The model under review builds one solid part; all positions refer to its coordinate system, in mm. A direction names the side the tool comes from. Coordinates: 2 decimals unless noted, no trailing zeros. Write each loop counter-clockwise with the first axis right and the second up, starting at its lowest first coordinate (ties: lowest second). Pieces come first, ordered by that corner, then holes. Notation, with made-up numbers: M 33,75.5 L 56,75.5 A12 ccw 56,92.5 Z; hole C 29.25,33.5 d5. An arc over 180 degrees is marked long. Answer as a JSON object with one key per item and string values.
```python
from build123d import *

# Parameters (mm, degrees)
CHANFREIN1_SIZE              = 0.5
ENL_V_MAT_EXTRU_1_DEPTH      = 8.95
ENL_V_MAT_EXTRU_1_DEPTH_BACK = 8.95


with BuildPart() as part:
    # Esquisse1 → Base-Révolution (revolve)
    with BuildSketch(Plane.XY, mode=Mode.PRIVATE) as base_r_volution_sk:
        with BuildLine():
            Line((0, 65), (4, 65))
            Line((4, 65), (4, 49))
            Line((4, 49), (6, 49))
            Line((6, 49), (6, 27))
            Line((6, 27), (7.95, 27))
            Line((7.95, 27), (7.95, 7.95))
            ThreePointArc((7.95, 7.95), (5.62149891, 2.32850109), (0, 0))
            Line((0, 0), (0, 65))
        make_face()
    revolve(base_r_volution_sk.sketch.rotate(Axis((0, -9.281443849, 0), (0, 1, 0)), 90), axis=Axis((0, -9.281443849, 0), (0, 1, 0)))  # turned: the seam where the file's is

    # Chanfrein1
    chanfrein1_edges = [part.edges().sort_by_distance(p)[0] for p in [
        (0, 65, 4),
    ]]
    chamfer(chanfrein1_edges, length=CHANFREIN1_SIZE)

    # Esquisse2 → Enlèv. mat.-Extru.1 (cut, two sides)
    with BuildSketch(Plane.XY) as enl_v_mat_extru_1_sk:
        Polygon((14.617538198, 1), (14.617538198, 10), (3.65, 10), (7.95, 21.8), (23.946768439, 21.8), (23.946768439, -11.083879123), (-11.532407151, -11.083879123), (-11.532407151, 1), align=None)
    extrude(amount=ENL_V_MAT_EXTRU_1_DEPTH, mode=Mode.SUBTRACT)
    extrude(enl_v_mat_extru_1_sk.sketch, amount=-ENL_V_MAT_EXTRU_1_DEPTH_BACK, mode=Mode.SUBTRACT)


solid = part.part
```
(1) Add section A-A on x = 0. Give the boundary of the cut face in (y, z), and give its area (3 significant figures).
Results list:
{"outline": "M 1,-3.86 A7.95 ccw 7.95,-7.95 L 27,-7.95 L 27,-6 L 49,-6 L 49,-4 L 64.5,-4 L 65,-3.5 L 65,3.5 L 64.5,4 L 49,4 L 49,6 L 27,6 L 27,7.95 L 7.95,7.95 A7.95 ccw 1,3.86 Z", "area": "789 mm²"}
(2) Add section C-C on y = 51.5. Give the boundary of the cut face in (x, z), and give its area (3 significant figures).
Results list:
{"outline": "C 0,0 d8", "area": "50.3 mm²"}
(3) For faces 4 (the face through (0, 65, 0)), 5 (the face through (-1.802, 37.846, -5.723)), list the 3-axis set-ups (+Z, -Z, +X, -X, +Y, -Y) from which the entire face can be reached by the end or side of a thin tool; tool diameter is ignored.
Results list:
{"face 4": "+Z, -Z, +X, -X, +Y", "face 5": "+Y"}
(4) Add section B-B on z = 0. Give the boundary of the cut face in (x, y), and give its area (3 significant figures).
Results list:
{"outline": "M -7.95,7.95 A7.95 ccw -3.86,1 L 3.86,1 A7.95 ccw 7.95,7.95 L 7.95,10 L 3.65,10 L 7.95,21.8 L 7.95,27 L 6,27 L 6,49 L 4,49 L 4,64.5 L 3.5,65 L -3.5,65 L -4,64.5 L -4,49 L -6,49 L -6,27 L -7.95,27 Z", "area": "763 mm²"}
(5) Wall thickness on line 1 along Z through (x, y) = (-5.25, 31); line 2 along X through (y, z) = (57, 0.75); line 3 along X through (y, z) = (22, 0.25): over which ranges is each line inside the solid? List them lowest first. Write a range as from..to.
Results list:
{"line 1": "-2.9..2.9", "line 2": "-3.93..3.93", "line 3": "-7.95..7.95"}
(6) For pin 1 Ø1.3 at (x, z) = (5.5, 0) entering from +Y; pin 2 Ø8 at (x, z) = (5.5, -5.5) entering from -Y; pin 3 Ø5 at (y, z) = (19, -4.5) entering from +X; pin 4 Ø2 at (y, z) = (18, -5) entering from +X, all flat-tipped, find the tip position at first contact; note any pin that passes through.
Results list:
{"pin 1": "y = 49", "pin 2": "y = 1", "pin 3": "x = 7.52", "pin 4": "x = 6.77"}
(7) Draft analysis for pull direction Y (two halves, no side actions). For faces 1 (the face through (5, 10, 0)), 2 (the face through (3.905, 56.642, 0.867)), 3 (the face through (3.92, 49, -1.42)), state which applies: released by +Y, released by -Y, zero draft, split by the parting line, or undercut.
Results list:
{"face 1": "undercut", "face 2": "zero draft", "face 3": "released by +Y"}
